Geometry check sheet. Reference: the model listing, model coordinates, mm. Face numbers are marked on the shaded views. A direction names the side the tool comes from. Coordinates: 2 decimals unless noted, no trailing zeros. Order: outer loops, then holes, each group sorted by start corner. A loop starts at its lowest first (then second) coordinate and runs counter-clockwise, first axis right, second up. Notation, with made-up numbers: (44.25, 61) - (91.25, 61) arc R19 cw to (91.25, 88) - close; hole circle Ø10 at (23.25, -36). An arc over 180 degrees is marked (long way). Put each result on its own line as item: value.
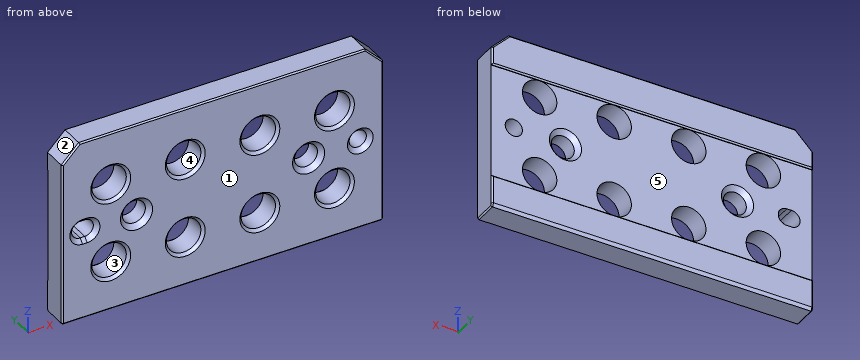
from build123d import *

# Parameters (mm, degrees)
EXTRUDE1_DEPTH                         = 88.9
EXTRUDE5_REACH                         = 90.9
EXTRUDE5_DIRECTION_2_REACH             = 90.9
F_3_4_0_75_DIAMETER_HOLE1_D            = 19.05
F_3_4_0_75_DIAMETER_HOLE1_DEPTH        = 18.5166
SKETCH6_W                              = 177.8
SKETCH6_H                              = 63.5
EXTRUDE2_DEPTH                         = 1.016
CHAMFER10_SIZE                         = 9.652
SKETCH35_W                             = 101.092
SKETCH35_H                             = 4.2926
EXTRUDE11_DEPTH                        = 89.9
EXTRUDE11_DEPTH_BACK                   = 89.9
F_3_8_0_375_DIAMETER_HOLE1_D           = 9.54278
F_3_8_0_375_DIAMETER_HOLE1_CSINK_D     = 14.224
F_3_8_0_375_DIAMETER_HOLE1_CSINK_ANGLE = 90
EXTRUDE8_DEPTH                         = 15.224
CHAMFER13_SIZE                         = 2.286
F_1_2_0_5_DIAMETER_HOLE4_AT_2_COUNT    = 2
F_1_2_0_5_DIAMETER_HOLE4_AT_2_PITCH    = 95.25
CHAMFER16_SIZE                         = 0.762
CHAMFER19_SIZE                         = 1.524


with BuildPart() as part:
    # Sketch1 → Extrude1 (new body, symmetric)
    with BuildSketch(Plane(origin=(0, 0, 0), x_dir=(0, 0, -1), z_dir=(1, 0, 0))):
        Polygon((-47.625, 0), (-51.435, 0), (-51.435, -18.5166), (-47.625, -18.5166), (47.625, -18.5166), (47.625, 0), align=None)
    extrude(amount=EXTRUDE1_DEPTH, both=True)

    # Extrude5: up to this face of the body (flat: up to its plane)
    extrude5_end = Plane(part.part.faces().sort_by_distance((-88.9, -9.2583, 1.905))[0])
    # Sketch10 → Extrude5 (add, up to the picked face)
    with BuildSketch(Plane(origin=(0, 0, 0), x_dir=(0, 0, -1), z_dir=(1, 0, 0)), mode=Mode.PRIVATE) as extrude5_sk1:
        with BuildLine():
            Line((47.625, 0), (47.625, -18.5166))
            Line((47.625, -18.5166), (49.657, -18.5166))
            Line((49.657, -18.5166), (49.657, -0.735409666))
            ThreePointArc((49.657, -0.735409666), (48.705491945, -0.189508055), (47.625, 0))
        make_face()
    extrude5_tool1 = split(extrude(extrude5_sk1.sketch, amount=-EXTRUDE5_REACH, mode=Mode.PRIVATE), bisect_by=extrude5_end, keep=Keep.BOTH, mode=Mode.PRIVATE)
    add(extrude5_tool1.solids().sort_by(Axis((0, -9.373301, -48.63438), (-1, 0, 0)))[0])

    # Extrude5 direction 2: up to this face of the body (flat: up to its plane)
    extrude5_direction_2_end = Plane(part.part.faces().sort_by_distance((88.9, -9.2583, 1.905))[0])
    # Sketch10 → Extrude5 direction 2 (add, up to the picked face)
    with BuildSketch(Plane(origin=(0, 0, 0), x_dir=(0, 0, -1), z_dir=(1, 0, 0)), mode=Mode.PRIVATE) as extrude5_direction_2_sk1:
        with BuildLine():
            Line((47.625, 0), (47.625, -18.5166))
            Line((47.625, -18.5166), (49.657, -18.5166))
            Line((49.657, -18.5166), (49.657, -0.735409666))
            ThreePointArc((49.657, -0.735409666), (48.705491945, -0.189508055), (47.625, 0))
        make_face()
    extrude5_direction_2_tool1 = split(extrude(extrude5_direction_2_sk1.sketch, amount=EXTRUDE5_DIRECTION_2_REACH, mode=Mode.PRIVATE), bisect_by=extrude5_direction_2_end, keep=Keep.BOTH, mode=Mode.PRIVATE)
    add(extrude5_direction_2_tool1.solids().sort_by(Axis((0, -9.373301, -48.63438), (1, 0, 0)))[0])

    # 3/4 (0.75) Diameter Hole1
    with Locations(Plane(origin=(100.583096031, 0, 72.51255066), x_dir=(-1, 0, 0), z_dir=(0, 1, 0))):
        with Locations((162.495596031, -94.73755066), (121.220596031, -94.73755066), (79.945596031, -94.73755066), (38.670596031, -94.73755066), (79.945596031, -50.28755066), (121.220596031, -50.28755066), (162.495596031, -50.28755066), (38.670596031, -50.28755066)):
            Hole(F_3_4_0_75_DIAMETER_HOLE1_D / 2, depth=F_3_4_0_75_DIAMETER_HOLE1_DEPTH)

    # Sketch6 → Extrude2 (cut)
    with BuildSketch(Plane(origin=(0, 0, 0), x_dir=(1, 0, 0), z_dir=(0, 1, 0))):
        Rectangle(SKETCH6_W, SKETCH6_H)
    extrude(amount=-EXTRUDE2_DEPTH, mode=Mode.SUBTRACT)

    # Chamfer10
    chamfer10_edges = [part.edges().sort_by_distance(p)[0] for p in [
        (88.9, -9.2583, 51.435),
        (-88.9, -9.2583, 51.435),
    ]]
    chamfer(chamfer10_edges, length=CHAMFER10_SIZE)

    # Sketch35 → Extrude11 (cut, two sides)
    with BuildSketch(Plane(origin=(0, 0, 0), x_dir=(0, 0, -1), z_dir=(1, 0, 0))) as extrude11_sk:
        with Locations((-0.889, -16.3703)):
            Rectangle(SKETCH35_W, SKETCH35_H)
    extrude(amount=EXTRUDE11_DEPTH, mode=Mode.SUBTRACT)
    extrude(extrude11_sk.sketch, amount=-EXTRUDE11_DEPTH_BACK, mode=Mode.SUBTRACT)

    # 3/8 (0.375) Diameter Hole1 (through all)
    with Locations(Plane(origin=(11.630068396, -14.224, 20.686230534), x_dir=(1, 0, 0), z_dir=(0, -1, 0))):
        with Locations((64.569931604, -20.686230534)):
            CounterSinkHole(F_3_8_0_375_DIAMETER_HOLE1_D / 2, F_3_8_0_375_DIAMETER_HOLE1_CSINK_D / 2, counter_sink_angle=F_3_8_0_375_DIAMETER_HOLE1_CSINK_ANGLE)

    # Sketch19 → Extrude8 (cut, through all)
    with BuildSketch(Plane.XZ.offset(14.224)):
        with BuildLine():
            Line((-77.47, 4.77139), (-74.93, 4.77139))
            ThreePointArc((-74.93, 4.77139), (-70.15861, 0), (-74.93, -4.77139))
            Line((-74.93, -4.77139), (-77.47, -4.77139))
            ThreePointArc((-77.47, -4.77139), (-82.24139, 0), (-77.47, 4.77139))
        make_face()
    extrude(amount=-EXTRUDE8_DEPTH, mode=Mode.SUBTRACT)

    # Chamfer13
    chamfer13_edges = [part.edges().sort_by_distance(p)[0] for p in [
        (-82.24139, -14.224, 0),
        (-76.2, -14.224, -4.77139),
        (-70.15861, -14.224, 0),
        (-76.2, -14.224, 4.77139),
    ]]
    chamfer(chamfer13_edges, length=CHAMFER13_SIZE)

    # Sketch26 → 1/2 (0.5) Diameter Hole4 (revolve, cut)
    with BuildSketch(Plane(origin=(-47.625, -1.016, 0), x_dir=(0, 0, 1), z_dir=(1, 0, 0))):
        Polygon((0, 0), (0, 13.208), (8.89, 13.208), (6.3754, 10.6934), (6.3754, 2.5146), (8.89, 0), align=None)
    f_1_2_0_5_diameter_hole4 = revolve(axis=Axis((-47.625, 5.334, 0), (0, -1, 0)), mode=Mode.SUBTRACT)

    # 1/2 (0.5) Diameter Hole4 at 2: 1/2 (0.5) Diameter Hole4 ×2
    with Locations(*[(i * F_1_2_0_5_DIAMETER_HOLE4_AT_2_PITCH, 0, 0) for i in range(1, F_1_2_0_5_DIAMETER_HOLE4_AT_2_COUNT)]):
        add(f_1_2_0_5_diameter_hole4, mode=Mode.SUBTRACT)

    # Chamfer16
    chamfer16_edges = [part.edges().sort_by_distance(p)[0] for p in [
        (0, 0, 31.75),
        (0, 0, -31.75),
        (88.9, 0, -39.6875),
        (0, 0, 51.435),
        (-84.074, 0, 46.609),
        (84.074, 0, 46.609),
        (-84.074, -14.224, 46.609),
        (88.9, -7.479704833, -49.657),
        (-88.9, -14.224, -3.937),
        (0, -14.224, 51.435),
        (84.074, -14.224, 46.609),
        (0, -14.224, -49.657),
        (88.9, -14.224, -3.937),
        (-88.9, -7.479704833, -49.657),
        (-88.9, -0.189508055, -48.705491945),
        (88.9, -0.189508055, -48.705491945),
        (-88.9, 0, -39.6875),
        (-88.9, 0, 36.7665),
        (88.9, 0, 36.7665),
    ]]
    chamfer(chamfer16_edges, length=CHAMFER16_SIZE)

    # Chamfer19
    chamfer19_edges = [part.edges().sort_by_distance(p)[0] for p in [
        (-71.4375, -14.224, 22.225),
        (11.1125, -14.224, 22.225),
        (11.1125, -14.224, -22.225),
        (-71.4375, -14.224, -22.225),
        (-30.1625, -14.224, -22.225),
        (52.3875, -14.224, -22.225),
        (-30.1625, -14.224, 22.225),
        (52.3875, -14.224, 22.225),
    ]]
    chamfer(chamfer19_edges, length=CHAMFER19_SIZE)


solid = part.part
Q1. Depth check by flat-ended pin: pin 1 Ø19 at (x, z) = (13.5, 5.5) entering from +Y. Enter the tip coordinate at first touch or a pass-through.
Answer block:
pin 1: stops at y = -1.02
Q2. Thickness scan on L1, parallel to X at y = -5.5, z = 0; L2, parallel to X at y = -4.25, z = 22.5; L3, parallel to Z at x = 62, y = -6.25 (3 decimals). Record the ranges inside material, lowest first. Write a range as [from, to].
Answer block:
L1: x = [-88.9, -82.24], [-70.16, -54], [-41.25, 41.25], [54, 71.43], [80.97, 88.9]
L2: x = [-88.9, -71.43], [-52.39, -30.16], [-11.12, 11.12], [30.16, 52.39], [71.43, 88.9]
L3: z = [-49.657, -31.75], [-12.7, 12.7], [31.75, 51.435]
Q3. Section check B-B on x = 76.2. Record the boundary of the cut face in (y, z) (3 decimals).
Answer block:
outline: (-14.224, -48.895) - (-13.462, -49.657) - (-0.735, -49.657) arc R3.175 ccw to (0, -47.625) - (0, -32.512) - (-0.762, -31.75) - (-1.016, -31.75) - (-1.016, -4.771) - (-11.883, -4.771) - (-14.224, -7.112) - close; (-14.224, 7.112) - (-11.883, 4.771) - (-1.016, 4.771) - (-1.016, 31.75) - (-0.762, 31.75) - (0, 32.512) - (0, 50.673) - (-0.762, 51.435) - (-13.462, 51.435) - (-14.224, 50.673) - close
Q4. Section check A-A on z = 0. State how many separate pieces and enclosed holes the cut face has, then the cut area to 3 significant figures.
Answer block:
separate pieces: 5
enclosed holes: 0
area: 1,690 mm^2
Q5. Draft check along X on the marked faces 1, 2 and 3. Enter one of: pulls with the +X half, pulls with the -X half, needs draft (parallel to the pull), parting line crosses it, or undercut.
Answer block:
face 1: needs draft
face 2: pulls with the -X half
face 3: undercut
Q6. Access from +Z, -Z, +X, -X, +Y, -Y to the whole of each face (thin tool, end or side, straight path). Record for the marked faces 4 and 5.
Answer block:
face 4: +Y, -Y
face 5: +X, -X, +Y
